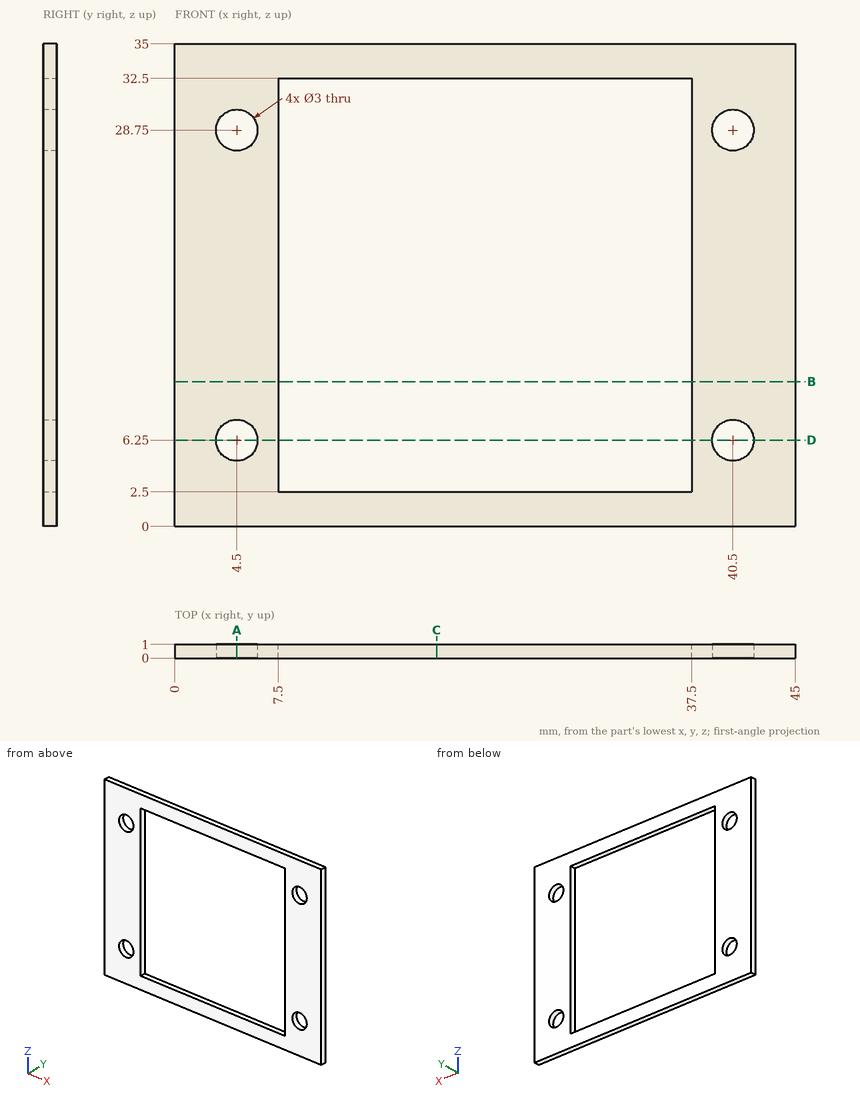
Geometry: see drawing. Coordinates: mm, zero at the bounding-box minimum. Coordinates: 2 decimals unless noted, no trailing zeros. Order: outer loops, then holes, each group sorted by start corner. A loop starts at its lowest first (then second) coordinate and runs counter-clockwise, first axis right, second up. Notation, with made-up numbers: M 36,31.25 L 42,31.25 A15 cw 42,46.25 Z; hole C -8.75,-5 d11. An arc over 180 degrees is marked long. Answer in a Markdown table with one row per item. Add a question column.
Q1. Section query C-C on x = 19. Return the cut outline in (y, z), and give its area (3 significant figures).
Q2. Section query D-D on z = 6.25. Return the cut outline in (x, y).
Q3. Line query: L1, parallel to X at y = 0.75, z = 6.25; L2, parallel to Z at x = 34, y = 0.55; L3, parallel to X at y = 0.2, z = 21. Output: solid intervals per line, ascending.
Q4. Section query B-B on z = 10.5. Return the cut outline in (x, y).
Q5. Section query A-A on x = 4.5. Return the cut outline in (y, z).
Completed:
| question | item | result |
|---|---|---|
| 1 | outline | M 0,0 L 1,0 L 1,2.5 L 0,2.5 Z; M 0,32.5 L 1,32.5 L 1,35 L 0,35 Z |
| 1 | area | 5.00 mm2 |
| 2 | outline | M 0,0 L 3,0 L 3,1 L 0,1 Z; M 6,0 L 7.5,0 L 7.5,1 L 6,1 Z; M 37.5,0 L 39,0 L 39,1 L 37.5,1 Z; M 42,0 L 45,0 L 45,1 L 42,1 Z |
| 3 | L1 | x = 0 to 3, 6 to 7.5, 37.5 to 39, 42 to 45 |
| 3 | L2 | z = 0 to 2.5, 32.5 to 35 |
| 3 | L3 | x = 0 to 7.5, 37.5 to 45 |
| 4 | outline | M 0,0 L 7.5,0 L 7.5,1 L 0,1 Z; M 37.5,0 L 45,0 L 45,1 L 37.5,1 Z |
| 5 | outline | M 0,0 L 1,0 L 1,4.75 L 0,4.75 Z; M 0,7.75 L 1,7.75 L 1,27.25 L 0,27.25 Z; M 0,30.25 L 1,30.25 L 1,35 L 0,35 Z |
